from build123d import *

# Parameters (mm, degrees)
SCHIZZO1_W                        = 720
SCHIZZO1_H                        = 620
ESTRUSIONE_ESTRUSIONE1_DEPTH      = 393
SCHIZZO3_W                        = 720
SCHIZZO3_H                        = 620
SCHIZZO3_W_2                      = 660
SCHIZZO3_H_2                      = 560
TAGLIO_ESTRUSIONE1_DEPTH          = 381
SCHIZZO4_R                        = 5.25
TAGLIO_ESTRUSIONE2_DEPTH          = 12
SCHIZZO5_W                        = 644
SCHIZZO5_H                        = 544
TAGLIO_ESTRUSIONE3_DEPTH          = 385
ESTRUSIONE_ESTRUSIONE2_DEPTH      = 10
ESTRUSIONE_ESTRUSIONE2_DEPTH_BACK = 20
SCHIZZO6_R                        = 125
SCHIZZO7_R                        = 90
TAGLIO_ESTRUSIONE4_DEPTH          = 30
FORO_PER_VITE_M10_1_D             = 11
RIPETIZIONECIRCOLARE1_COUNT       = 6
SCHIZZO14_W                       = 600
SCHIZZO14_H                       = 300
TAGLIO_ESTRUSIONE5_DEPTH          = 8
SCHIZZO16_R                       = 5.25
TAGLIO_ESTRUSIONE6_DEPTH          = 8
TAGLIO_ESTRUSIONE7_START          = -8
SCHIZZO17_R                       = 5.25
TAGLIO_ESTRUSIONE7_DEPTH          = 8
SCHIZZO18_W                       = 272
SCHIZZO18_H                       = 220
TAGLIO_ESTRUSIONE8_DEPTH          = 8
SCHIZZO19_W                       = 200
SCHIZZO19_H                       = 160
ESTRUSIONE_ESTRUSIONE3_DEPTH      = 12
SCHIZZO20_W                       = 45
SCHIZZO20_H                       = 11
TAGLIO_ESTRUSIONE9_DEPTH          = 20


with BuildPart() as part:
    # Schizzo1 → Estrusione-Estrusione1 (new body)
    with BuildSketch(Plane(origin=(0, 0, 0), x_dir=(1, 0, 0), z_dir=(0, 1, 0))):
        with Locations((360, 310)):
            Rectangle(SCHIZZO1_W, SCHIZZO1_H)
    extrude(amount=ESTRUSIONE_ESTRUSIONE1_DEPTH)

    # Schizzo3 → Taglio-Estrusione1 (cut)
    with BuildSketch(Plane(origin=(0, 393, 0), x_dir=(1, 0, 0), z_dir=(0, 1, 0))):
        with Locations((360, 310)):
            Rectangle(SCHIZZO3_W, SCHIZZO3_H)
        with Locations((360, 310)):
            Rectangle(SCHIZZO3_W_2, SCHIZZO3_H_2, mode=Mode.SUBTRACT)
    extrude(amount=-TAGLIO_ESTRUSIONE1_DEPTH, mode=Mode.SUBTRACT)

    # Schizzo4 → Taglio-Estrusione2 (cut)
    with BuildSketch(Plane(origin=(0, 12, 0), x_dir=(1, 0, 0), z_dir=(0, 1, 0))):
        with Locations(Location((360, 605, 0), (0, 0, 270))):
            Circle(SCHIZZO4_R)
        with Locations(Location((650, 605, 0), (0, 0, 270))):
            Circle(SCHIZZO4_R)
        with Locations(Location((70, 605, 0), (0, 0, 90))):
            Circle(SCHIZZO4_R)
        with Locations(Location((650, 15, 0), (0, 0, 90))):
            Circle(SCHIZZO4_R)
        with Locations(Location((360, 15, 0), (0, 0, 90))):
            Circle(SCHIZZO4_R)
        with Locations(Location((70, 15, 0), (0, 0, 270))):
            Circle(SCHIZZO4_R)
        with Locations(Location((705, 560, 0), (0, 0, 270))):
            Circle(SCHIZZO4_R)
        with Locations(Location((705, 290, 0), (0, 0, 270))):
            Circle(SCHIZZO4_R)
        with Locations(Location((705, 50, 0), (0, 0, 270))):
            Circle(SCHIZZO4_R)
        with Locations(Location((15, 50, 0), (0, 0, 90))):
            Circle(SCHIZZO4_R)
        with Locations(Location((15, 290, 0), (0, 0, 90))):
            Circle(SCHIZZO4_R)
        with Locations(Location((15, 560, 0), (0, 0, 90))):
            Circle(SCHIZZO4_R)
    extrude(amount=-TAGLIO_ESTRUSIONE2_DEPTH, mode=Mode.SUBTRACT)

    # Schizzo5 → Taglio-Estrusione3 (cut)
    with BuildSketch(Plane(origin=(0, 0, 0), x_dir=(1, 0, 0), z_dir=(0, 1, 0))):
        with Locations((360, 310)):
            Rectangle(SCHIZZO5_W, SCHIZZO5_H)
    extrude(amount=TAGLIO_ESTRUSIONE3_DEPTH, mode=Mode.SUBTRACT)

    # Schizzo6 → Estrusione-Estrusione2 (add, two sides: drawn at the far end of the back side and taken through both)
    with BuildSketch(Plane(origin=(0, 393, 0), x_dir=(1, 0, 0), z_dir=(0, 1, 0)).offset(-ESTRUSIONE_ESTRUSIONE2_DEPTH_BACK)):
        with Locations(Location((360, 290, 0), (0, 0, 270))):
            Circle(SCHIZZO6_R)
    extrude(amount=ESTRUSIONE_ESTRUSIONE2_DEPTH + ESTRUSIONE_ESTRUSIONE2_DEPTH_BACK)

    # Schizzo7 → Taglio-Estrusione4 (cut)
    with BuildSketch(Plane(origin=(0, 403, 0), x_dir=(1, 0, 0), z_dir=(0, 1, 0))):
        with Locations(Location((360, 290, 0), (0, 0, 270))):
            Circle(SCHIZZO7_R)
    extrude(amount=-TAGLIO_ESTRUSIONE4_DEPTH, mode=Mode.SUBTRACT)

    # Foro per Vite M10-1 (through all)
    with Locations(Plane(origin=(465, 403, -290), x_dir=(0, 0, 1), z_dir=(0, 1, 0))):
        with Locations((0, 0)):
            foro_per_vite_m10_1 = Hole(FORO_PER_VITE_M10_1_D / 2)

    # RipetizioneCircolare1: Foro per Vite M10-1 ×6 about axis
    ripetizionecircolare1_axis = Axis((360, 0, -290), (0, 1, 0))
    for i in range(1, RIPETIZIONECIRCOLARE1_COUNT):
        add(foro_per_vite_m10_1.rotate(ripetizionecircolare1_axis, i * 360 / RIPETIZIONECIRCOLARE1_COUNT), mode=Mode.SUBTRACT)

    # Schizzo14 → Taglio-Estrusione5 (cut)
    with BuildSketch(Plane.XY.offset(-582)):
        with Locations((360, 190)):
            Rectangle(SCHIZZO14_W, SCHIZZO14_H)
    extrude(amount=-TAGLIO_ESTRUSIONE5_DEPTH, mode=Mode.SUBTRACT)

    # Schizzo16 → Taglio-Estrusione6 (cut)
    with BuildSketch(Plane.ZY.offset(-30)):
        with Locations((-310, 90)):
            Circle(SCHIZZO16_R)
        with Locations((-270, 90)):
            Circle(SCHIZZO16_R)
    extrude(amount=-TAGLIO_ESTRUSIONE6_DEPTH, mode=Mode.SUBTRACT)

    # Schizzo17 → Taglio-Estrusione7 (cut)
    with BuildSketch(Plane(origin=(690, 0, 0), x_dir=(0, 0, -1), z_dir=(1, 0, 0)).offset(TAGLIO_ESTRUSIONE7_START)):
        with Locations(Location((310, 90, 0), (0, 0, 180))):
            Circle(SCHIZZO17_R)
        with Locations(Location((270, 90, 0), (0, 0, 180))):
            Circle(SCHIZZO17_R)
    extrude(amount=TAGLIO_ESTRUSIONE7_DEPTH, mode=Mode.SUBTRACT)

    # Schizzo18 → Taglio-Estrusione8 (cut)
    with BuildSketch(Plane.ZY.offset(-682)):
        with Locations((-174, 275)):
            Rectangle(SCHIZZO18_W, SCHIZZO18_H)
    extrude(amount=-TAGLIO_ESTRUSIONE8_DEPTH, mode=Mode.SUBTRACT)

    # Schizzo19 → Estrusione-Estrusione3 (add)
    with BuildSketch(Plane(origin=(0, 0, -38), x_dir=(-1, 0, 0), z_dir=(0, 0, -1))):
        with Locations((-582, 272)):
            Rectangle(SCHIZZO19_W, SCHIZZO19_H)
    extrude(amount=ESTRUSIONE_ESTRUSIONE3_DEPTH)

    # Schizzo20 → Taglio-Estrusione9 (cut)
    with BuildSketch(Plane(origin=(0, 0, -50), x_dir=(-1, 0, 0), z_dir=(0, 0, -1))):
        with Locations((-624, 216.5)):
            Rectangle(SCHIZZO20_W, SCHIZZO20_H)
        with Locations((-529, 216.5)):
            Rectangle(SCHIZZO20_W, SCHIZZO20_H)
        with Locations((-529, 327.5)):
            Rectangle(SCHIZZO20_W, SCHIZZO20_H)
        with Locations((-624, 327.5)):
            Rectangle(SCHIZZO20_W, SCHIZZO20_H)
    extrude(amount=-TAGLIO_ESTRUSIONE9_DEPTH, mode=Mode.SUBTRACT)


solid = part.part
For this review, take the finished solid that the model builds, in its own axes (mm). A direction names the side the tool comes from. Coordinates: 2 decimals unless noted, no trailing zeros. Loops run counter-clockwise (first coordinate to the right, second up) from the corner with the lowest first, then second, coordinate; pieces in that order, holes last. Notation, with made-up numbers: (88.5, 46) - (116.5, 46) arc R13 ccw to (116.5, 68) - close; hole circle Ø9 at (0.5, 67). An arc over 180 degrees is marked (long way). Return JSON: item names as keys, results as strings.
Item 1: Take a section at B-B (x = 207). Give the boundary of the cut face in (y, z).
Determined:
{"outline": "(0, -620) - (12, -620) - (12, -590) - (40, -590) - (40, -582) - (0, -582) - close; (0, -38) - (385, -38) - (385, -582) - (340, -582) - (340, -590) - (393, -590) - (393, -30) - (12, -30) - (12, 0) - (0, 0) - close"}
Item 2: For line 1 (X direction, y = 7.5, z = -50); line 2 (X direction, y = 2, z = -15); line 3 (Z direction, x = 39.5, y = 61), list the stretches that pass through material, from the lowest coordinate up.
Determined:
{"line 1": "x = 0 to 9.75, 20.25 to 38, 682 to 699.75, 710.25 to 720", "line 2": "x = 0 to 64.75, 75.25 to 354.75, 365.25 to 644.75, 655.25 to 720", "line 3": "z = -590 to -582, -38 to -30"}
Item 3: Mouldability with a two-part tool opening along Y and no side actions: class faces 1 (the flat face through (624, 211, -40)), 2 (the flat face through (583, 273, -50)), 3 (the flat face through (277, 373, -254)) as pulls with the +Y half, pulls with the -Y half, needs draft (parallel to the pull), parting line crosses it, or undercut.
Determined:
{"face 1": "undercut", "face 2": "needs draft", "face 3": "pulls with the -Y half"}
Item 4: Take a section at C-C (z = -149). Give the boundary of the cut face in (x, y), then the cut area to 3 significant figures.
Determined:
{"outline": "(0, 0) - (38, 0) - (38, 385) - (690, 385) - (690, 393) - (30, 393) - (30, 12) - (0, 12) - close; (682, 0) - (720, 0) - (720, 12) - (690, 12) - (690, 165) - (682, 165) - close", "area": "10,400 mm2"}
Item 5: Take a section at A-A (y = 263). Give the boundary of the cut face in (x, z).
Determined:
{"outline": "(30, -590) - (60, -590) - (60, -582) - (38, -582) - (38, -38) - (482, -38) - (482, -50) - (682, -50) - (682, -38) - (690, -38) - (690, -30) - (30, -30) - close; (660, -590) - (690, -590) - (690, -310) - (682, -310) - (682, -582) - (660, -582) - close"}
Item 6: Take a section at D-D (x = 395). Give the boundary of the cut face in (y, z), then the cut area to 3 significant figures.
Determined:
{"outline": "(0, -620) - (12, -620) - (12, -590) - (40, -590) - (40, -582) - (0, -582) - close; (0, -38) - (385, -38) - (385, -170) - (373, -170) - (373, -207.08) - (403, -207.08) - (403, -170) - (393, -170) - (393, -30) - (12, -30) - (12, 0) - (0, 0) - close; (340, -590) - (393, -590) - (393, -410) - (403, -410) - (403, -372.92) - (373, -372.92) - (373, -410) - (385, -410) - (385, -582) - (340, -582) - close", "area": "9,270 mm2"}
Item 7: Insertion check: pin 1 (5.5 mm diameter, centred on y = 219, z = -36, fed in from +X); pin 2 (9 mm diameter, centred on y = 325, z = -44, fed in from -X); pin 3 (1 mm diameter, centred on x = 613, z = -234.5, fed in from +Y). Each pin has a flat end and moves straight along its axis. Give the tip position at first contact, or say it passes through.
Determined:
{"pin 1": "stops at x = 690", "pin 2": "stops at x = 30", "pin 3": "stops at y = 393"}
Item 8: For faces 4 (the flat face through (30, 205, -306)), 5 (the flat face through (624, 333, -40)), 6 (the cylindrical face through (397.547, 378.916, -170.772)), 7 (the cylindrical face through (397.547, 397.93, -170.772)), list the 3-axis set-ups (+Z, -Z, +X, -X, +Y, -Y) from which the entire face can be reached by the end or side of a thin tool; tool diameter is ignored.
Determined:
{"face 4": "+Z, -Z, -X, +Y", "face 5": "+Z, -Z", "face 6": "-Y", "face 7": "+Y"}
